Could you check a few things on this drawing? It's one solid part, dimensions in mm from its lowest x, y, z. Give positions to 0.01 mm unless a question says otherwise; leave off trailing zeros. Write each loop counter-clockwise with the first axis right and the second up, starting at its lowest first coordinate (ties: lowest second). Pieces come first, ordered by that corner, then holes. Notation, with made-up numbers: (-27.5, 17.5) - (-5.5, 17.5) arc R20 cw to (-5.5, 41.5) - close; hole circle Ø8 at (42.25, -31). An arc over 180 degrees is marked (long way). One line per item, written item: value. Start each with the question number.
1) Imagine slicing it at C-C on x = 4. Write out the boundary of the cut face in (y, z).
2) I'm going to push a flat-ended pin straight in: P1, Ø2.5, axis at x = 34, y = 4, coming from the +Z side. Where does the tip first touch, or does it pass through?
3) Please list where these lines run through material, in increasing order: L1, parallel to X at y = 16, z = 1; L2, parallel to Y at x = 4, z = 1.6; L3, parallel to X at y = 29, z = 1.35. Write a range as [from, to].
4) Imagine slicing it at B-B on z = 1.55. Write out the boundary of the cut face in (x, y).
5) Imagine slicing it at A-A on y = 16. Write out the boundary of the cut face in (x, z).
6) Imagine slicing it at D-D on y = 29. Write out the boundary of the cut face in (x, z), plus the area to 3 significant figures.
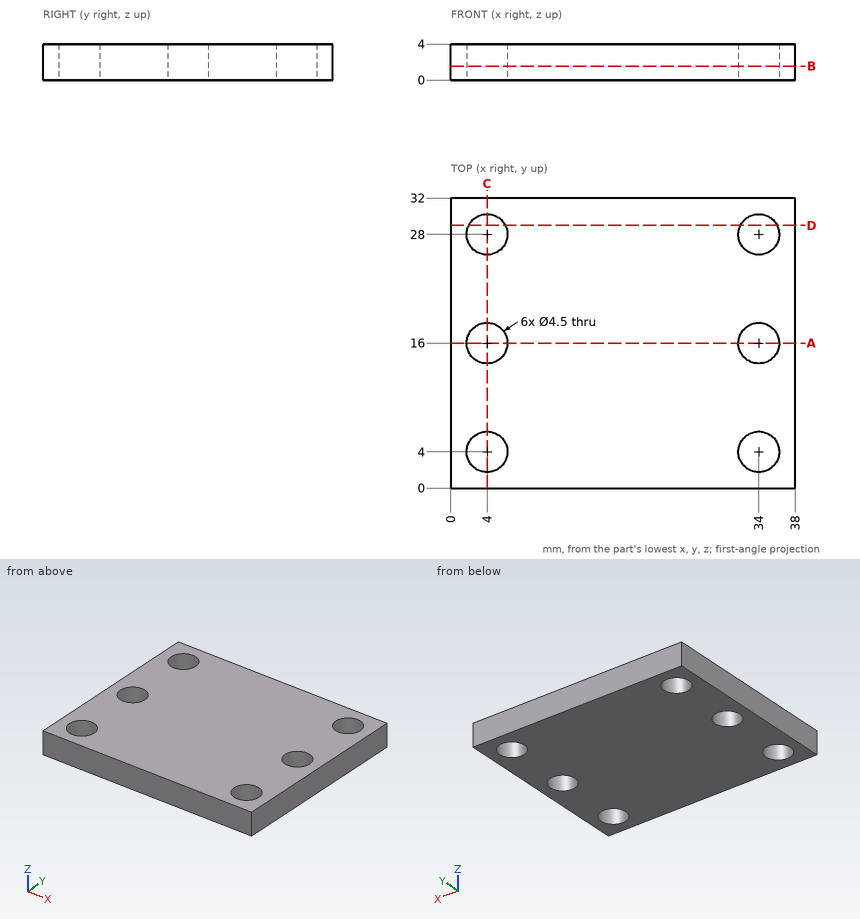
Numbers:
1. outline: (0, 0) - (1.75, 0) - (1.75, 4) - (0, 4) - close; (6.25, 0) - (13.75, 0) - (13.75, 4) - (6.25, 4) - close; (18.25, 0) - (25.75, 0) - (25.75, 4) - (18.25, 4) - close; (30.25, 0) - (32, 0) - (32, 4) - (30.25, 4) - close
2. P1: through
3. L1: [0, 1.75], [6.25, 31.75], [36.25, 38]
3. L2: [0, 1.75], [6.25, 13.75], [18.25, 25.75], [30.25, 32]
3. L3: [0, 1.98], [6.02, 31.98], [36.02, 38]
4. outline: (0, 0) - (38, 0) - (38, 32) - (0, 32) - close; hole circle Ø4.5 at (4, 4); hole circle Ø4.5 at (4, 16); hole circle Ø4.5 at (4, 28); hole circle Ø4.5 at (34, 4); hole circle Ø4.5 at (34, 16); hole circle Ø4.5 at (34, 28)
5. outline: (0, 0) - (1.75, 0) - (1.75, 4) - (0, 4) - close; (6.25, 0) - (31.75, 0) - (31.75, 4) - (6.25, 4) - close; (36.25, 0) - (38, 0) - (38, 4) - (36.25, 4) - close
6. outline: (0, 0) - (1.98, 0) - (1.98, 4) - (0, 4) - close; (6.02, 0) - (31.98, 0) - (31.98, 4) - (6.02, 4) - close; (36.02, 0) - (38, 0) - (38, 4) - (36.02, 4) - close
6. area: 120 mm^2
